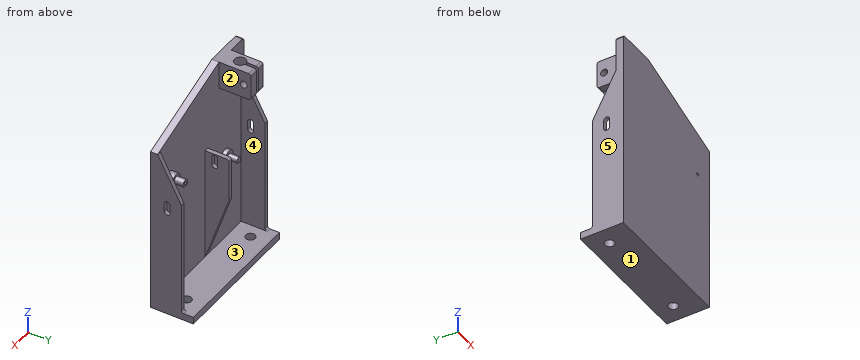
```python
from build123d import *

# Parameters (mm, degrees)
SKETCH1_W                               = 115
SKETCH1_H                               = 170
BACK_WALL_EXTRUDE_DEPTH                 = 6
SKETCH2_W                               = 115
SKETCH2_H                               = 6
BOTTOM_PLATE_EXTRUDE_DEPTH              = 30
SKETCH3_W                               = 3.5
SKETCH3_H                               = 135
SKETCH3_H_2                             = 96
SIDE_WALLS_EXTRUDE_DEPTH                = 20
SKETCH4_W                               = 16.3
SKETCH4_H                               = 23.5
DIAL_INDIACTOR_HOLDER_EXTRUDE_DEPTH     = 26.7
DIAL_INDICATOR_HOLE_CUT_DEPTH           = 26.7
SKETCH6_R                               = 3
DIAL_INDICATOR_TIGHTENER_HOLE_CUT_DEPTH = 26.7
SKETCH7_R                               = 5.1
ARM_BASE_EXTRUDE_DEPTH                  = 5.7
SKETCH8_R                               = 3
ARM_AXLE_EXTRUDE_DEPTH                  = 7.6
SKETCH9_R                               = 5.1
GUIDE_WHEEL_BASE_EXTRUDE_DEPTH          = 3.5
SKETCH10_R                              = 2.45
GUIDE_WHEEL_AXLE_EXTRUDE_DEPTH          = 8
FILAMENT_START                          = 71.967294703
FILAMENT_SLOT_CUT_OUTLINE_W             = 100
FILAMENT_SLOT_CUT_OUTLINE_H             = 6
FILAMENT_SLOT_CUT_DEPTH                 = 27.34055864
FILAMENT_START_2                        = -115
FILAMENT_SLOT_CUT_2_DEPTH               = 116
SKETCH13_R                              = 3.96875
MOUNTING_HOLES_CUT_DEPTH                = 8
FILLET1_R                               = 2
CUT_EXTRUDE9_DEPTH                      = 8
SKETCH15_R                              = 1.225
SCREW_HOLE_CUT_DEPTH                    = 105.420974904
CUT_EXTRUDE11_DEPTH                     = 148.465250144


with BuildPart() as part:
    # Sketch1 → Back Wall Extrude (new body)
    with BuildSketch(Plane(origin=(0, 0, 0), x_dir=(1, 0, 0), z_dir=(0, 1, 0))):
        Rectangle(SKETCH1_W, SKETCH1_H)
    extrude(amount=BACK_WALL_EXTRUDE_DEPTH)

    # Sketch2 → Bottom Plate Extrude (add)
    with BuildSketch(Plane(origin=(0, 6, 0), x_dir=(1, 0, 0), z_dir=(0, 1, 0))):
        with Locations((0, 82)):
            Rectangle(SKETCH2_W, SKETCH2_H)
    extrude(amount=BOTTOM_PLATE_EXTRUDE_DEPTH)

    # Sketch3 → Side Walls Extrude (add)
    with BuildSketch(Plane(origin=(0, 6, 0), x_dir=(1, 0, 0), z_dir=(0, 1, 0))):
        with Locations((-55.75, 11.5)):
            Rectangle(SKETCH3_W, SKETCH3_H)
        with Locations((55.75, 11.5)):
            Rectangle(SKETCH3_W, SKETCH3_H)
        with Locations((-7.75, 31)):
            Rectangle(SKETCH3_W, SKETCH3_H_2)
    extrude(amount=SIDE_WALLS_EXTRUDE_DEPTH)

    # Sketch4 → Dial Indiactor Holder Extrude (add)
    with BuildSketch(Plane(origin=(0, 6, 0), x_dir=(1, 0, 0), z_dir=(0, 1, 0))):
        with Locations((-32.65, -73.25)):
            Rectangle(SKETCH4_W, SKETCH4_H)
    extrude(amount=DIAL_INDIACTOR_HOLDER_EXTRUDE_DEPTH)

    # Sketch5 → Dial Indicator Hole Cut (cut)
    with BuildSketch(Plane.XY.offset(85)):
        with BuildLine():
            Line((-34.538403692, 32.7), (-32.038403692, 32.7))
            Line((-32.038403692, 32.7), (-32.038403692, 22.762553146))
            ThreePointArc((-32.038403692, 22.762553146), (-33.433435972, 13.450573614), (-34.538403692, 22.801409096))
            Line((-34.538403692, 22.801409096), (-34.538403692, 32.7))
        make_face()
    extrude(amount=-DIAL_INDICATOR_HOLE_CUT_DEPTH, mode=Mode.SUBTRACT)

    # Sketch6 → Dial Indicator Tightener Hole Cut (cut)
    with BuildSketch(Plane.ZY.offset(40.8)):
        with Locations((73.25, 26.7)):
            Circle(SKETCH6_R)
    extrude(amount=-DIAL_INDICATOR_TIGHTENER_HOLE_CUT_DEPTH, mode=Mode.SUBTRACT)

    # Sketch7 → Arm Base Extrude (add)
    with BuildSketch(Plane(origin=(0, 6, 0), x_dir=(1, 0, 0), z_dir=(0, 1, 0))):
        with Locations(Location((41.6, -24.9, 0), (0, 0, 90))):
            Circle(SKETCH7_R)
    extrude(amount=ARM_BASE_EXTRUDE_DEPTH)

    # Sketch8 → Arm Axle Extrude (add)
    with BuildSketch(Plane(origin=(0, 11.7, 0), x_dir=(1, 0, 0), z_dir=(0, 1, 0))):
        with Locations(Location((41.6, -24.9, 0), (0, 0, 90))):
            Circle(SKETCH8_R)
    extrude(amount=ARM_AXLE_EXTRUDE_DEPTH)

    # Sketch9 → Guide Wheel Base Extrude (add)
    with BuildSketch(Plane(origin=(0, 6, 0), x_dir=(1, 0, 0), z_dir=(0, 1, 0))):
        with Locations(Location((-32.6, 4.4, 0), (0, 0, 90))):
            Circle(SKETCH9_R)
    extrude(amount=GUIDE_WHEEL_BASE_EXTRUDE_DEPTH)

    # Sketch10 → Guide Wheel Axle Extrude (add)
    with BuildSketch(Plane(origin=(0, 9.5, 0), x_dir=(1, 0, 0), z_dir=(0, 1, 0))):
        with Locations(Location((-32.6, 4.4, 0), (0, 0, 270))):
            Circle(SKETCH10_R)
    extrude(amount=GUIDE_WHEEL_AXLE_EXTRUDE_DEPTH)

    # Filament Slot Cut: read off the stored shape, not the designer's step
    # Filament Slot Cut outline → Filament Slot Cut (cut)
    with BuildSketch(Plane(origin=(0, 0, 0), x_dir=(0.942777884125997, 0, -0.333421446825048), z_dir=(0.333421446825048, 0, 0.942777884125997)).offset(FILAMENT_START)):
        with Locations((-3, 3)):
            Rectangle(FILAMENT_SLOT_CUT_OUTLINE_W, FILAMENT_SLOT_CUT_OUTLINE_H)
    extrude(amount=FILAMENT_SLOT_CUT_DEPTH, mode=Mode.SUBTRACT)

    # Filament Slot Cut 2 outline → Filament Slot Cut 2 (cut)
    with BuildSketch(Plane.ZY.offset(57.5).offset(FILAMENT_START_2)):
        with BuildLine():
            ThreePointArc((14, 11.51558642), (16.5, 14.01558642), (14, 16.51558642))
            Line((14, 16.51558642), (7, 16.51558642))
            ThreePointArc((7, 16.51558642), (4.5, 14.01558642), (7, 11.51558642))
            Line((7, 11.51558642), (14, 11.51558642))
        make_face()
    extrude(amount=FILAMENT_SLOT_CUT_2_DEPTH, mode=Mode.SUBTRACT)

    # Sketch13 → Mounting Holes Cut (cut)
    with BuildSketch(Plane(origin=(0, 0, -85), x_dir=(-1, 0, 0), z_dir=(0, 0, -1))):
        with Locations((42.5, 21)):
            Circle(SKETCH13_R)
        with Locations((-42.5, 21)):
            Circle(SKETCH13_R)
    extrude(amount=-MOUNTING_HOLES_CUT_DEPTH, mode=Mode.SUBTRACT)

    # Fillet1
    fillet1_edges = [part.edges().sort_by_distance(p)[0] for p in [
        (-55.75, 26, 56),
        (-55.75, 26, -79),
        (55.75, 26, -79),
        (55.75, 26, 56),
        (-7.75, 26, 17),
        (-37.669201846, 32.7, 85),
        (-28.269201846, 32.7, 61.5),
        (-57.5, 3, 85),
        (-28.269201846, 32.7, 85),
        (-37.669201846, 32.7, 61.5),
    ]]
    fillet(fillet1_edges, radius=FILLET1_R)

    # Sketch14 → Cut-Extrude9 (cut)
    with BuildSketch(Plane.ZY.offset(9.5)):
        Polygon((-79, 6), (-19.585405324, 26), (-79, 26), align=None)
    extrude(amount=-CUT_EXTRUDE9_DEPTH, mode=Mode.SUBTRACT)

    # Sketch15 → Screw Hole Cut (cut, through all)
    with BuildSketch(Plane(origin=(0, 19.3, 0), x_dir=(1, 0, 0), z_dir=(0, 1, 0))):
        with Locations(Location((41.6, -24.9, 0), (0, 0, 270))):
            Circle(SKETCH15_R)
    extrude(amount=-SCREW_HOLE_CUT_DEPTH, mode=Mode.SUBTRACT)

    # Sketch16 → Cut-Extrude11 (cut, through all)
    with BuildSketch(Plane.ZY.offset(57.5)):
        Polygon((56, 6), (17.948284572, 26), (56, 26), align=None)
    extrude(amount=-CUT_EXTRUDE11_DEPTH, mode=Mode.SUBTRACT)


solid = part.part
```
Geometry: final body of the model. Coordinates: model frame, mm. Face numbers are marked on the shaded views. A direction names the side the tool comes from. Coordinates: 2 decimals unless noted, no trailing zeros. Loops run counter-clockwise (first coordinate to the right, second up) from the corner with the lowest first, then second, coordinate; pieces in that order, holes last. Notation, with made-up numbers: (64, -20.5) -> (89, -20.5) arc R25 cw to (89, 17.5) -> close; hole circle Ø7 at (-33.5, 67). An arc over 180 degrees is marked (long way). Use a Markdown table: item, result. Add a question column.
(1) Pin query (flat end, axial travel): pin 1 Ø1 at (x, y) = (22, 10) entering from +Z; pin 2 Ø3 at (x, z) = (55, 10) entering from +Y; pin 3 Ø5 at (x, z) = (42, 24.5) entering from +Y; pin 4 Ø10 at (x, z) = (-18.5, 41.5) entering from -Y. Return the tip coordinate at first contact, or that it passes through.
(2) Section query C-C, the plane x = -49. Return loops of the section in (y, z).
(3) Section query A-A, the plane z = 73.25. Return loops of the section in (x, y).
(4) Section query D-D, the plane z = 43.5. Return loops of the section in (x, y), plus the area to 3 significant figures.
(5) Access query for the marked faces 4 and 5. Directions: +Z, -Z, +X, -X, +Y, -Y. A direction counts if a zero-diameter tool reaches every point of the face in a straight line with its end or side. Return the directions, or none.
(6) Section query B-B, the plane y = 3. Return loops of the section in (x, z) (3 decimals).
(7) Mould query, pull axis X, two halves, no side actions, for the marked faces 1, 2 and 3. Classes: pulls with the +X half, pulls with the -X half, needs draft (parallel to the pull), parting line crosses it, or undercut.
(8) Line query: line 1 along X through (y, z) = (10.5, -58); line 2 along Y through (x, z) = (42, -80); line 3 along Z through (x, y) = (-26, 26). Output: solid intervals per line, ascending.
Answer:
| question | item | result |
|---|---|---|
| 1 | pin 1 | stops at z = -79 |
| 1 | pin 2 | stops at y = 26 |
| 1 | pin 3 | stops at y = 19.3 |
| 1 | pin 4 | stops at y = 0 |
| 2 | outline | (0, -85) -> (36, -85) -> (36, -79) -> (6, -79) -> (6, 85) -> (0, 85) -> close |
| 3 | outline | (-57.5, 0) -> (8.72, 0) -> (8.72, 6) -> (-24.5, 6) -> (-24.5, 23.7) -> (-32.04, 23.7) -> (-32.04, 22.76) arc R4.75 cw (long way) to (-34.54, 22.8) -> (-34.54, 23.7) -> (-40.8, 23.7) -> (-40.8, 6) -> (-57.5, 6) -> close; (-40.8, 29.7) -> (-34.54, 29.7) -> (-34.54, 32.7) -> (-40.8, 32.7) -> close; (-32.04, 29.7) -> (-24.5, 29.7) -> (-24.5, 32.7) -> (-32.04, 32.7) -> close |
| 4 | outline | (-57.5, 0) -> (57.5, 0) -> (57.5, 12.57) -> (54, 12.57) -> (54, 6) -> (-54, 6) -> (-54, 12.57) -> (-57.5, 12.57) -> close |
| 4 | area | 736 mm^2 |
| 5 | face 4 | +Z, +Y |
| 5 | face 5 | +Z, -Z, -X, +Y, -Y |
| 6 | outline | (-57.5, -85) -> (57.5, -85) -> (57.5, 56) -> (-24.5, 85) -> (-55.5, 85) arc R2 ccw to (-57.5, 83) -> close; hole circle Ø2.45 at (41.6, 24.9) |
| 7 | face 1 | needs draft |
| 7 | face 2 | pulls with the +X half |
| 7 | face 3 | undercut |
| 8 | line 1 | x = -57.5 to -54, -9.5 to -6, 54 to 57.5 |
| 8 | line 2 | y = 0 to 17.06, 24.94 to 36 |
| 8 | line 3 | z = -85 to -79, 61.5 to 70.33, 76.17 to 85 |
